Study the drawing (mm; zero at the part's minimum x, y, z) and answer. A direction names the side the tool comes from. Give positions to 0.01 mm unless a question says otherwise; leave off trailing zeros. Loops run counter-clockwise (first coordinate to the right, second up) from the corner with the lowest first, then second, coordinate; pieces in that order, holes last. Notation, with made-up numbers: (-29, -15.75) -> (-7, -15.75) arc R21 cw to (-7, -8.75) -> close; hole circle Ø9 at (60.25, 9.25). An arc over 180 degrees is marked (long way). One line per question, with ' | ' between items. Start each with the question number.
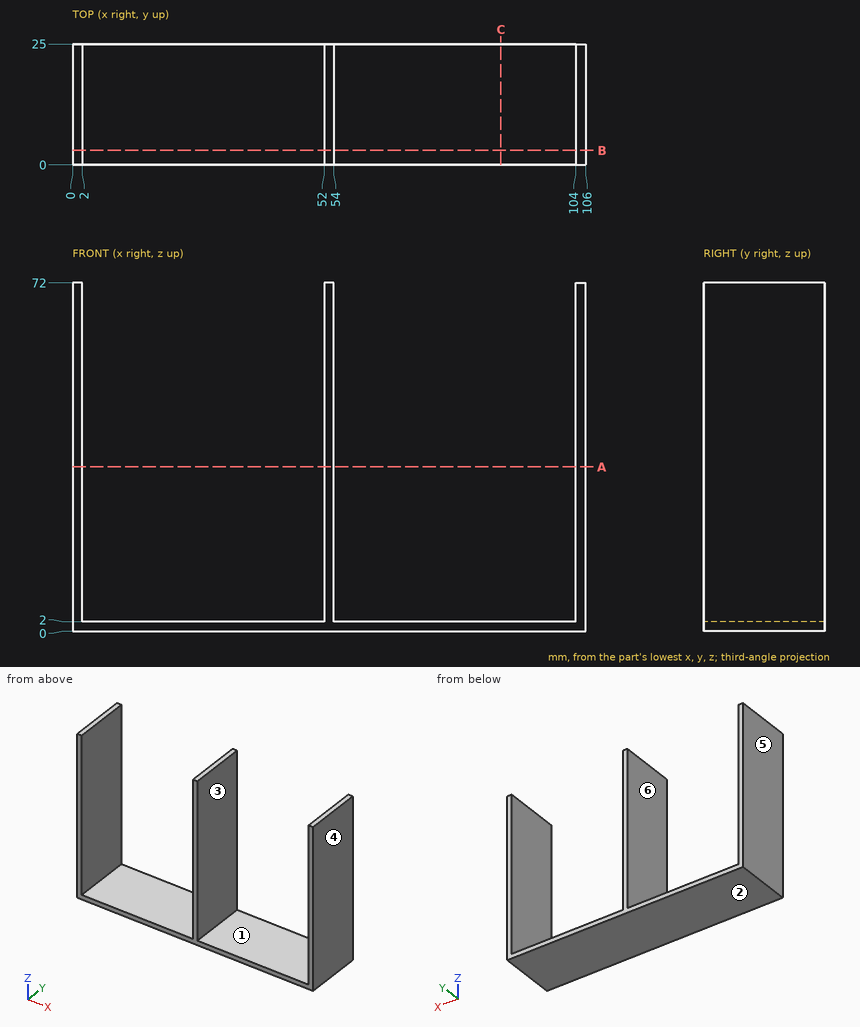
1. The part is cut by section A-A (z = 34). Write down the section's boundary in (x, y).
2. The part is cut by section B-B (y = 3). Write down the section's boundary in (x, z).
3. Determine the mould class of the marked faces 3, 4, 5 and 6 for opening direction X: released by +X, released by -X, zero draft, split by the parting line, or undercut.
4. This flat-tipped pin is pushed along its axis until it touches: pin 1 Ø7.5 at (x, y) = (37.5, 16) entering from +Z. Where does it stop, or does it pass through?
5. The part is cut by section C-C (x = 88.5). Write down the section's boundary in (y, z), plus the area to 3 significant figures.
6. For the marked faces 1 and 2, determine the directions among +Z, -Z, +X, -X, +Y, -Y from which every point of the face is accessible in a straight line to the end or side of a thin tool.
7. Straight lines are drawn through the part: L1, parallel to X at y = 18.75, z = 5.5; L2, parallel to Z at x = 26, y = 13. For each, find the intervals that lie inside material, in ascending order.
Check sheet entries:
1) outline: (0, 0) -> (2, 0) -> (2, 25) -> (0, 25) -> close; (52, 0) -> (54, 0) -> (54, 25) -> (52, 25) -> close; (104, 0) -> (106, 0) -> (106, 25) -> (104, 25) -> close
2) outline: (0, 0) -> (106, 0) -> (106, 72) -> (104, 72) -> (104, 2) -> (54, 2) -> (54, 72) -> (52, 72) -> (52, 2) -> (2, 2) -> (2, 72) -> (0, 72) -> close
3) face 3: undercut | face 4: released by +X | face 5: released by -X | face 6: undercut
4) pin 1: stops at z = 2
5) outline: (0, 0) -> (25, 0) -> (25, 2) -> (0, 2) -> close | area: 50.0 mm^2
6) face 1: +Z, +Y, -Y | face 2: -Z, +X, -X, +Y, -Y
7) L1: x = 0 to 2, 52 to 54, 104 to 106 | L2: z = 0 to 2
